The listing builds one solid part. Answer for the finished solid, in the listing's coordinates (mm). A direction names the side the tool comes from. Coordinates: 2 decimals unless noted, no trailing zeros. Write each loop counter-clockwise with the first axis right and the second up, starting at its lowest first coordinate (ties: lowest second). Pieces come first, ordered by that corner, then holes. Notation, with made-up numbers: M 69.5,80.25 L 128.5,80.25 A27 ccw 128.5,117.25 Z; hole C 54,22 d3. An arc over 180 degrees is marked long. Answer as a JSON object with one key per item and string values. Group by question number.
from build123d import *

# Parameters (mm, degrees)
F1_DEPTH      = 25
F2_W          = 45
F2_H          = 45
F3_DEPTH      = 615
F4_W          = 45
F4_H          = 45
F5_DEPTH      = 287
F5_DEPTH_BACK = 615
F6_W          = 25
F6_H          = 80
F6_H_2        = 36
F7_DEPTH      = 135
F7_DEPTH_BACK = 155
F8_W          = 25
F8_H          = 80
F8_H_2        = 30
F9_DEPTH      = 155
F9_DEPTH_BACK = 155
F12_DEPTH     = 32.5
F14_DEPTH     = 10


with BuildPart() as f1:
    # F0 (on Top) → F1 (new body)
    with BuildSketch(Plane.XY):
        with BuildLine():
            Line((155, 200), (-155, 200))
            Line((-155, 200), (-155, 155))
            Line((-155, 155), (-200, 155))
            Line((-200, 155), (-200, -160))
            ThreePointArc((-200, -160), (-188.2842712475, -188.2842712475), (-160, -200))
            Line((-160, -200), (160, -200))
            ThreePointArc((160, -200), (188.2842712475, -188.2842712475), (200, -160))
            Line((200, -160), (200, 155))
            Line((200, 155), (155, 155))
            Line((155, 155), (155, 200))
        make_face()
    extrude(amount=F1_DEPTH)

    # F2 (on Top) → F3 (join)
    with BuildSketch(Plane.XY):
        with Locations((157.5, -157.5)):
            Rectangle(F2_W, F2_H)
        with Locations((-157.5, -157.5)):
            Rectangle(F2_W, F2_H)
    extrude(amount=-F3_DEPTH)

    # F4 (on Top) → F5 (join, two sides)
    with BuildSketch(Plane.XY) as f5_sk:
        with Locations((-177.5, 177.5)):
            Rectangle(F4_W, F4_H)
        with Locations((177.5, 177.5)):
            Rectangle(F4_W, F4_H)
    extrude(amount=F5_DEPTH)
    extrude(f5_sk.sketch, amount=-F5_DEPTH_BACK)

    # F6 (on Front) → F7 (join, two sides)
    with BuildSketch(Plane.XZ) as f7_sk:
        with Locations((-167.5, -40)):
            Rectangle(F6_W, F6_H)
        with Locations((167.5, -40)):
            Rectangle(F6_W, F6_H)
        with Locations((-167.5, -378)):
            Rectangle(F6_W, F6_H_2)
        with Locations((167.5, -378)):
            Rectangle(F6_W, F6_H_2)
    extrude(amount=F7_DEPTH)
    extrude(f7_sk.sketch, amount=-F7_DEPTH_BACK)

    # F8 (on Right) → F9 (join, two sides)
    with BuildSketch(Plane.YZ) as f9_sk:
        with Locations((-157.5, -40)):
            Rectangle(F8_W, F8_H)
        with Locations((177.5, -40)):
            Rectangle(F8_W, F8_H)
        with Locations((-157.5, -456)):
            Rectangle(F8_W, F8_H_2)
    extrude(amount=F9_DEPTH)
    extrude(f9_sk.sketch, amount=-F9_DEPTH_BACK)

    # F11 (on offset) → F12 (join, symmetric)
    with BuildSketch(Plane.XZ.offset(-175)):
        with BuildLine():
            Line((210, 287), (-210, 287))
            ThreePointArc((-210, 287), (-233.0940107676, 273.6666666667), (-233.0940107676, 247))
            Line((-233.0940107676, 247), (-210, 207))
            Line((-210, 207), (210, 207))
            Line((210, 207), (233.0940107676, 247))
            ThreePointArc((233.0940107676, 247), (233.0940107676, 273.6666666667), (210, 287))
        make_face()
    extrude(amount=F12_DEPTH, both=True)

    # F13 (on offset) → F14 (join, symmetric)
    with BuildSketch(Plane.XZ.offset(-175)):
        Polygon((-155, 75), (-155, 50), (0, 111), (-31.762295082, 123.5), align=None)
        Polygon((-31.762295082, 123.5), (0, 111), (31.762295082, 123.5), (0, 136), align=None)
        Polygon((31.762295082, 123.5), (0, 111), (155, 50), (155, 75), align=None)
        Polygon((0, 136), (31.762295082, 123.5), (155, 172), (155, 197), align=None)
        Polygon((-155, 172), (-31.762295082, 123.5), (0, 136), (-155, 197), align=None)
    extrude(amount=F14_DEPTH, both=True)


solid = f1.part
Item 1: A cutting plane is placed at D-D, the plane z = 63. Write down the section's boundary in (x, y).
Item 2: Flat-ended cylindrical pins translate along their axes: pin 1 Ø1 at (x, y) = (12.5, 90) entering from -Z; pin 2 Ø20 at (x, y) = (-173.5, -59.5) entering from +Z; pin 3 Ø24 at (x, z) = (-6.5, -450.5) entering from +Y. Find the tip coordinate at first contact, or state that the pin passes through.
Item 3: A cutting plane is placed at A-A, the plane z = -417. Write down the section's boundary in (x, y).
Item 4: A cutting plane is placed at B-B, the plane y = -114. Write down the section's boundary in (x, z).
Item 5: For a pull along Y with two mould halves and no side action, classify faces 1 (the face through (167, 12, -396)), 2 (the face through (-1, 185, 118)), 3 (the face through (-168, 12, -396)), 4 (the face through (200, 166, -145)) as +Y half, -Y half, draft (parallel to the pull), parting line (faces both ways), or undercut.
Item 6: A tool of negligible diameter and unlimited length cuts with its end or side. For faces 5 (the face through (2, -145, -41)), 6 (the face through (155, 177, 115)), 7 (the face through (76.415, 174.86, 80.927)), from which of +Z, -Z, +X, -X, +Y, -Y can it reach the whole face along a straight path? Write none if from no direction.
Item 7: A cutting plane is placed at C-C, the plane x = -88. Write down the section's boundary in (y, z).
Item 8: Consider L1, parallel to Z at x = -162.5, y = 153; L2, parallel to X at y = -114.5, z = -1; L3, parallel to Z at x = 171.5, y = 44. Determine where each line is inside the solid, lowest interval first. Write a range as from..to.
Answer:
{
 "1": {"outline": "M -200,155 L -155,155 L -155,165 L -121.97,165 L -121.97,185 L -155,185 L -155,200 L -200,200 Z; M 121.97,165 L 155,165 L 155,155 L 200,155 L 200,200 L 155,200 L 155,185 L 121.97,185 Z"},
 "2": {"pin 1": "z = 0", "pin 2": "z = 25", "pin 3": "y = -145"},
 "3": {"outline": "M -200,155 L -155,155 L -155,200 L -200,200 Z; M -180,-180 L -135,-180 L -135,-135 L -180,-135 Z; M 135,-180 L 180,-180 L 180,-135 L 135,-135 Z; M 155,155 L 200,155 L 200,200 L 155,200 Z"},
 "4": {"outline": "M -200,0 L -180,0 L -180,-80 L -155,-80 L -155,0 L 155,0 L 155,-80 L 180,-80 L 180,0 L 200,0 L 200,25 L -200,25 Z; M -180,-396 L -155,-396 L -155,-360 L -180,-360 Z; M 155,-396 L 180,-396 L 180,-360 L 155,-360 Z"},
 "5": {"face 1": "undercut", "face 2": "+Y half", "face 3": "undercut", "face 4": "draft"},
 "6": {"face 5": "-Z", "face 6": "none", "face 7": "+Y, -Y"},
 "7": {"outline": "M -200,0 L -170,0 L -170,-80 L -145,-80 L -145,0 L 165,0 L 165,-80 L 190,-80 L 190,0 L 200,0 L 200,25 L -200,25 Z; M -170,-471 L -145,-471 L -145,-441 L -170,-441 Z; M 142.5,207 L 207.5,207 L 207.5,287 L 142.5,287 Z; M 165,76.37 L 185,76.37 L 185,101.37 L 165,101.37 Z; M 165,145.63 L 185,145.63 L 185,170.63 L 165,170.63 Z"},
 "8": {"L1": "-396..-360, -80..25, 207..287", "L2": "-180..-155, 155..180", "L3": "-396..-360, -80..25"}
}
